Could you check a few things on this model? Use its own coordinates, in mm. Round coordinates to 2 decimals unless told otherwise and drop trailing zeros. Write each loop counter-clockwise with the first axis right and the second up, starting at its lowest first coordinate (ties: lowest second). Pieces come first, ordered by that corner, then holes. Notation, with made-up numbers: (44.25, -5) -> (59.25, -5) arc R33 ccw to (59.25, 28) -> close; hole circle Ø11 at (34, -34.75). An arc over 180 degrees is marked (long way). One line per question, with ' | ' between items. Start each with the question number.
1. Imagine slicing it at A-A, the plane z = 38.1. List the corners of the cut face in (x, y) for me (3 decimals), and give its area (3 significant figures).
2. Imagine slicing it at D-D, the plane y = -2.35. State how many separate pieces and enclosed holes the cut face has, and give its area (3 significant figures).
3. Imagine slicing it at C-C, the plane z = 0. List the corners of the cut face in (x, y) for me (3 decimals), and give its area (3 significant figures).
4. For pin 1 Ø2.5 at (x, z) = (-50.8, 12.7) entering from -Y; pin 2 Ø1.6 at (x, y) = (-4, -1) entering from +Z, each with a flat end and sliding along its axis, tell me the tip position at first contact or that it passes through.
5. If I drill on line 1 along Z through (x, y) = (51, -2.3); line 2 along X through (y, z) = (-2.7, 11.5); line 3 along X through (y, z) = (-2.75, -25), over which ranges is the centre line in solid material (lowest first)? Write a range as [from, to].
6. Imagine slicing it at B-B, the plane x = -88.9. List the corners of the cut face in (y, z) for me (3 decimals).
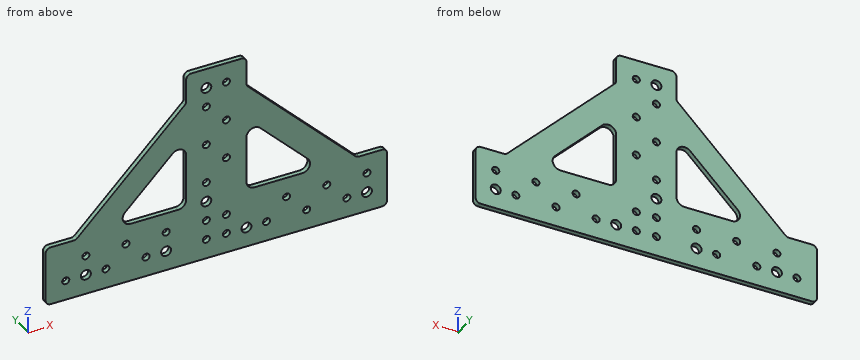
from build123d import *

# Parameters (mm, degrees)
F1_DEPTH = 3.175
F2_R     = 3.175
F3_R     = 5.08
F5_D     = 6.35
F6_D     = 4.4958
F7_R     = 5.08


with BuildPart() as f1:
    # F0 (on Front) → F1 (new body)
    with BuildSketch(Plane.XZ):
        Polygon((-25.4, 63.5), (-63.5, 63.5), (-63.5, 44.45), (-133.35, -25.4), (-152.4, -25.4), (-152.4, -63.5), (-63.5, -63.5), (63.5, -63.5), (63.5, -25.4), (44.45, -25.4), (-25.4, 44.45), align=None)
        Polygon((-63.5, 21.9964), (-63.5, -25.4), (-110.8964, -25.4), align=None, mode=Mode.SUBTRACT)
        Polygon((-25.4, -25.4), (-25.4, 21.9993596973), (21.9993596973, -25.4), align=None, mode=Mode.SUBTRACT)
    extrude(amount=F1_DEPTH)

    # F2
    f2_edges = [f1.edges().sort_by_distance(p)[0] for p in [
        (-25.4, -1.5875, 63.5),
        (-25.4, -1.5875, 44.45),
        (44.45, -1.5875, -25.4),
        (63.5, -1.5875, -25.4),
        (63.5, -1.5875, -63.5),
        (-63.5, -1.5875, 63.5),
        (-133.35, -1.5875, -25.4),
        (-152.4, -1.5875, -25.4),
        (-152.4, -1.5875, -63.5),
        (-63.5, -1.5875, 44.45),
    ]]
    fillet(f2_edges, radius=F2_R)

    # F3
    f3_edges = [f1.edges().sort_by_distance(p)[0] for p in [
        (21.99936, -1.5875, -25.4),
        (-25.4, -1.5875, -25.4),
        (-25.4, -1.5875, 21.99936),
    ]]
    fillet(f3_edges, radius=F3_R)

    # F5 (through all)
    with Locations(Plane.XZ.offset(3.175)):
        with Locations((-50.8, 50.8), (-50.8, -25.4), (50.8, -50.8), (-25.4, -50.8), (-76.2, -50.8), (-127, -50.8)):
            Hole(F5_D / 2)

    # F6 (through all)
    with Locations(Plane.XZ.offset(3.175)):
        with Locations((-50.8, 38.1), (-38.1, 50.8), (-38.1, 25.4), (-50.8, 12.7), (-38.1, 0), (-50.8, -12.7), (-38.1, -38.1), (-50.8, -38.1), (-50.8, -50.8), (-38.1, -50.8), (-12.7, -50.8), (0, -38.1), (12.7, -50.8), (25.4, -38.1), (38.1, -50.8), (50.8, -38.1), (-139.7, -50.8), (-127, -38.1), (-114.3, -50.8), (-101.6, -38.1), (-88.9, -50.8), (-76.2, -38.1)):
            Hole(F6_D / 2)

    # F7
    f7_edges = [f1.edges().sort_by_distance(p)[0] for p in [
        (-110.8964, -1.5875, -25.4),
        (-63.5, -1.5875, -25.4),
        (-63.5, -1.5875, 21.9964),
    ]]
    fillet(f7_edges, radius=F7_R)


solid = f1.part
Geometry results:
1) outline: (-69.85, -3.175) -> (-53.048, -3.175) -> (-53.048, 0) -> (-69.85, 0) -> close; (-48.552, -3.175) -> (-19.05, -3.175) -> (-19.05, 0) -> (-48.552, 0) -> close | area: 147 mm2
2) separate pieces: 1 | enclosed holes: 30 | area: 13,800 mm2
3) outline: (-107.95, -3.175) -> (-85.496, -3.175) -> (-85.496, 0) -> (-107.95, 0) -> close; (-63.5, -3.175) -> (-40.348, -3.175) -> (-40.348, 0) -> (-63.5, 0) -> close; (-35.852, -3.175) -> (-25.4, -3.175) -> (-25.4, 0) -> (-35.852, 0) -> close; (-3.401, -3.175) -> (19.05, -3.175) -> (19.05, 0) -> (-3.401, 0) -> close | area: 249 mm2
4) pin 1: passes through | pin 2: stops at z = 23.85
5) line 1: z = [-63.5, -53.97], [-47.63, -40.34], [-35.86, -25.4] | line 2: x = [-96.45, -74], [-63.82, -52.7], [-48.9, -25.08], [-14.9, 7.55] | line 3: x = [-133.12, -100.61], [-66.6, -53.95], [-47.65, -22.3], [11.71, 44.22]
6) outline: (-3.175, -63.5) -> (0, -63.5) -> (0, -53.048) -> (-3.175, -53.048) -> close; (-3.175, -48.552) -> (0, -48.552) -> (0, -25.4) -> (-3.175, -25.4) -> close; (-3.175, -3.404) -> (0, -3.404) -> (0, 19.05) -> (-3.175, 19.05) -> close
